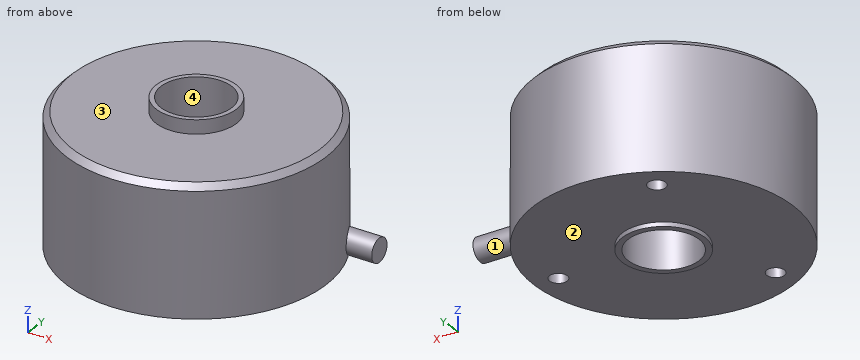
Autodesk Inventor part; units mm, degrees
ref_plane "YZ Plane" through (0, 0, 0) normal (1, 0, 0) x (0, 1, 0)
ref_plane "XZ Plane" through (0, 0, 0) normal (0, 1, 0) x (-1, 0, 0)
ref_plane "XY Plane" through (0, 0, 0) normal (0, 0, 1) x (1, 0, 0)
sketch "スケッチ1" plane through (0, 0, 0) normal (0, 0, 1) x (1, 0, 0)
  circle A0 centre (0, 0) radius 22
  dimension "d0" = 44
extrude "押し出し1" add sketch "スケッチ1" along normal blind 21.9
chamfer "面取り1" distance 1 angle 45 1 edges at (-22, 0, 21.9)
sketch "スケッチ2" plane through (0, 0, 21.9) normal (0, 0, 1) x (1, 0, 0)
  circle A0 centre (0, 0) radius 6.8
  dimension "d6" = 13.6
extrude "押し出し2" add sketch "スケッチ2" along normal blind 2.35
sketch "スケッチ6" plane through (0, 0, 0) normal (0, 0, 1) x (1, 0, 0)
  point P0 (0, 0)
sketch "スケッチ8" plane through (0, 0, 0) normal (0, 1, 0) x (-1, 0, 0)
  point P0 (0, 0)
sketch "スケッチ9" plane through (0, 0, 0) normal (1, 0, 0) x (0, 1, 0)
  line L0 (-22, 0) -> (22, 0)
  circle A0 centre (9.6776, 2.25) radius 2
  point P0 (0, 0)
  dimension "d30" = 2.25
  dimension "d31" = 4
extrude "押し出し3" add sketch "スケッチ9" along normal blind 25
sketch "スケッチ12" plane through (0, 0, 0) normal (0, 0, -1) x (-1, 0, 0)
  circle A0 centre (0, 0) radius 7
  dimension "d44" = 14
extrude "押し出し5" add sketch "スケッチ12" along normal blind 0.75
sketch "スケッチ13" plane through (0, 0, 24.25) normal (0, 0, 1) x (1, 0, 0)
  point P0 (0, 0)
  point P1 (0, 0)
hole "穴4" at (0, 0, 24.25) direction (0, 0, -1) diameter 12 end through all
sketch "スケッチ14" plane through (0, 0, 0) normal (0, 0, -1) x (-1, 0, 0)
  point P0 (0, 0)
  point P1 (-18, 0)
  point P2 (9, -15.5885)
  point P3 (9, 15.5885)
  dimension "d54" = 18
  dimension "d57" = 360
hole "穴5" at (18, 0, 0) at (-9, -15.5885, 0) at (-9, 15.5885, 0) direction (0, 0, 1) diameter 3 depth 5 tip angle 118
properties part number "meh-30-pエンコーダ"
Build history of the part. All positions in model axes, mm. Face numbers are marked on the shaded views. A direction names the side the tool comes from. Round coordinates to 2 decimals unless told otherwise and drop trailing zeros. Loops run counter-clockwise (first coordinate to the right, second up) from the corner with the lowest first, then second, coordinate; pieces in that order, holes last.
Item 1: Saw through at A-A (x = 0). List the corners of the cut face in (y, z).
Item 2: Drill centre lines: line 1 along Y through (x, z) = (0, 18); line 2 along Z through (x, y) = (-1.5, 17); line 3 along Y through (x, z) = (-9, 3.3). Where is each one in solid material? Low to high.
Item 3: Which spindle directions (+Z, -Z, +X, -X, +Y, -Y) get a long thin tool onto all of the face, cutting with end or side? Do the marked faces 1 and 2. Say none if no direction does.
Item 4: Two-plate mould, pull along Y, no slides. Class the marked faces 3 and 4: released by +Y, released by -Y, zero draft, split by the parting line, or undercut.
Item 5: Saw through at B-B (z = 2.25). List the corners of the cut face in (x, y).
Item 6: Saw through at C-C (z = 19.75). List the corners of the cut face in (x, y).
Item 7: Pin check, flat tips, straight feed: P1, Ø3, axis at x = 15, y = 4.5, coming from the +Z side; P2, Ø12, axis at x = -3, y = 17, coming from the -Z side; P3, Ø6, axis at y = -15.5, z = 21, coming from the -X side. Stop position of each tip, or through.
Worked answers:
1. outline: (-22, 0) - (-7, 0) - (-7, -0.75) - (-6, -0.75) - (-6, 24.25) - (-6.8, 24.25) - (-6.8, 21.9) - (-21, 21.9) - (-22, 20.9) - close; (6, -0.75) - (7, -0.75) - (7, 0) - (22, 0) - (22, 20.9) - (21, 21.9) - (6.8, 21.9) - (6.8, 24.25) - (6, 24.25) - close
2. line 1: y = -22 to -6, 6 to 22
2. line 2: z = 0 to 21.9
2. line 3: y = -20.07 to -17.09, -14.09 to 14.09, 17.09 to 20.07
3. face 1: +X
3. face 2: -Z
4. face 3: zero draft
4. face 4: undercut
5. outline: (18.64, 11.68) arc R22 ccw (long way) to (20.62, 7.68) - (25, 7.68) - (25, 11.68) - close; hole circle Ø3 at (-9, -15.59); hole circle Ø3 at (-9, 15.59); hole circle Ø12 at (0, 0); hole circle Ø3 at (18, 0)
6. outline: circle Ø44 at (0, 0); hole circle Ø12 at (0, 0)
7. P1: stops at z = 21.9
7. P2: stops at z = 0
7. P3: stops at x = -18.1
